Geometry check sheet. Reference: the model listing, model coordinates, mm. Face numbers are marked on the shaded views. A direction names the side the tool comes from. Give positions to 0.01 mm unless a question says otherwise; leave off trailing zeros. Loops run counter-clockwise (first coordinate to the right, second up) from the corner with the lowest first, then second, coordinate; pieces in that order, holes last.
1. Cross-section at C-C, the plane z = 0. Record the cut outline in (x, y).
2. Release check for a two-part mould opening along X. For the marked faces 1, 2 and 3 record: +X half, -X half, draft (parallel to the pull), parting line (faces both ways), or undercut.
3. Cross-section at D-D, the plane y = 52. Record the cut outline in (x, z), plus the area to 3 significant figures.
4. Tool access check on the marked faces 4, 5, 6 and 7. Record the directions out of +Z, -Z, +X, -X, +Y, -Y that give a thin tool (end or side, any length) a straight path to the whole face; none if there is none.
5. Cross-section at A-A, the plane y = 17. Record the cut outline in (x, z).
6. Cross-section at B-B, the plane x = -76.2. Record the cut outline in (y, z), plus the area to 3 significant figures.
7. Go/stop test with flat-tipped pins: pin 1 Ø8 at (y, z) = (21.5, 15.5) entering from +X; pin 2 Ø10 at (y, z) = (45.5, 15) entering from -X; pin 3 Ø1.5 at (x, y) = (57.5, 8) entering from -Z; pin 4 Ø5 at (x, z) = (-60, 14.5) entering from -Y. Record where each tip stops, or that it passes through.
8. Material ranges on L1, parallel to X at y = 28.5, z = 0; L2, parallel to X at y = 37, z = 0; L3, parallel to Z at x = -76, y = 28, recorded low to high.
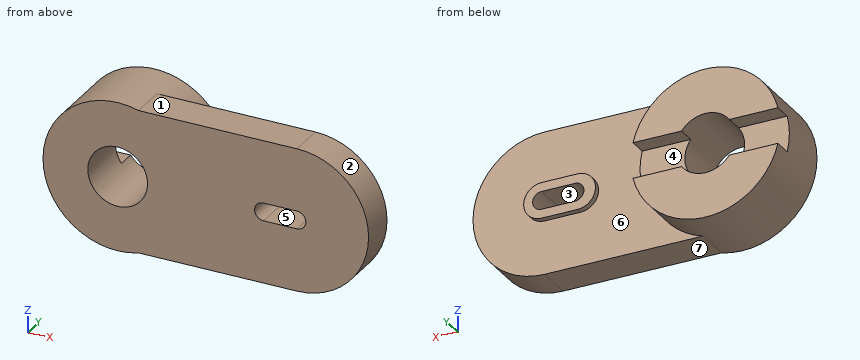
from build123d import *

# Parameters (mm, degrees)
SKETCH2_W           = 152.4
SKETCH2_H           = 121.92
BOSS_EXTRUDE1_DEPTH = 30.48
SKETCH3_R           = 63.5
BOSS_EXTRUDE2_DEPTH = 30.48
SKETCH4_R           = 25.4
CUT_EXTRUDE1_DEPTH  = 60.96
BOSS_EXTRUDE3_DEPTH = 30.48
BOSS_EXTRUDE5_DEPTH = 5.08
CUT_EXTRUDE4_DEPTH  = 35.56
CUT_EXTRUDE5_DEPTH  = 15.24


with BuildPart() as part:
    # Sketch2 → Boss-Extrude1 (new body)
    with BuildSketch(Plane(origin=(0, 0, 0), x_dir=(1, 0, 0), z_dir=(0, 1, 0))):
        Rectangle(SKETCH2_W, SKETCH2_H)
    extrude(amount=BOSS_EXTRUDE1_DEPTH)

    # Sketch3 → Boss-Extrude2 (add, symmetric)
    with BuildSketch(Plane(origin=(0, 30.48, 0), x_dir=(1, 0, 0), z_dir=(0, 1, 0))):
        with Locations(Location((-76.2, 0, 0), (0, 0, 73.739795292))):
            Circle(SKETCH3_R)
    extrude(amount=BOSS_EXTRUDE2_DEPTH, both=True)

    # Sketch4 → Cut-Extrude1 (cut)
    with BuildSketch(Plane(origin=(0, 60.96, 0), x_dir=(1, 0, 0), z_dir=(0, 1, 0))):
        with Locations(Location((-76.2, 0, 0), (0, 0, 270))):
            Circle(SKETCH4_R)
    extrude(amount=-CUT_EXTRUDE1_DEPTH, mode=Mode.SUBTRACT)

    # Sketch5 → Boss-Extrude3 (add)
    with BuildSketch(Plane(origin=(0, 30.48, 0), x_dir=(1, 0, 0), z_dir=(0, 1, 0))):
        with BuildLine():
            Line((76.2, 60.96), (76.2, -60.96))
            ThreePointArc((76.2, -60.96), (137.16, 0), (76.2, 60.96))
        make_face()
    extrude(amount=-BOSS_EXTRUDE3_DEPTH)

    # Sketch6 → Boss-Extrude5 (add)
    with BuildSketch(Plane(origin=(0, 30.48, 0), x_dir=(1, 0, 0), z_dir=(0, 1, 0))):
        with BuildLine():
            Line((76.2, -15.24), (45.597337332, -15.24))
            ThreePointArc((45.597337332, -15.24), (30.357337332, 0), (45.597337332, 15.24))
            Line((45.597337332, 15.24), (76.2, 15.24))
            ThreePointArc((76.2, 15.24), (91.44, 0), (76.2, -15.24))
        make_face()
    extrude(amount=BOSS_EXTRUDE5_DEPTH)

    # Sketch12 → Cut-Extrude4 (cut)
    with BuildSketch(Plane(origin=(0, 35.56, 0), x_dir=(1, 0, 0), z_dir=(0, 1, 0))):
        with BuildLine():
            Line((76.2, -7.62), (47.846010547, -7.62))
            ThreePointArc((47.846010547, -7.62), (40.226010547, 0), (47.846010547, 7.62))
            Line((47.846010547, 7.62), (76.2, 7.62))
            ThreePointArc((76.2, 7.62), (83.82, 0), (76.2, -7.62))
        make_face()
    extrude(amount=-CUT_EXTRUDE4_DEPTH, mode=Mode.SUBTRACT)

    # Sketch14 → Cut-Extrude5 (cut)
    with BuildSketch(Plane(origin=(0, 60.96, 0), x_dir=(1, 0, 0), z_dir=(0, 1, 0))):
        with BuildLine():
            Line((-137.844078386, -15.24), (-14.555921614, -15.24))
            ThreePointArc((-14.555921614, -15.24), (-12.7, 0), (-14.555921614, 15.24))
            Line((-14.555921614, 15.24), (-137.844078386, 15.24))
            ThreePointArc((-137.844078386, 15.24), (-139.7, 0), (-137.844078386, -15.24))
        make_face()
    extrude(amount=-CUT_EXTRUDE5_DEPTH, mode=Mode.SUBTRACT)


solid = part.part
Result:
1. outline: (-139.7, 0) - (-101.6, 0) - (-101.6, 45.72) - (-139.7, 45.72) - close; (-50.8, 0) - (40.23, 0) - (40.23, 35.56) - (30.36, 35.56) - (30.36, 30.48) - (-12.7, 30.48) - (-12.7, 45.72) - (-50.8, 45.72) - close; (83.82, 0) - (137.16, 0) - (137.16, 30.48) - (91.44, 30.48) - (91.44, 35.56) - (83.82, 35.56) - close
2. face 1: draft
2. face 2: +X half
2. face 3: undercut
3. outline: (-137.84, -15.24) arc R63.5 ccw to (-14.56, -15.24) - (-55.88, -15.24) arc R25.4 cw to (-96.52, -15.24) - close; (-137.84, 15.24) - (-96.52, 15.24) arc R25.4 cw to (-55.88, 15.24) - (-14.56, 15.24) arc R63.5 ccw to start
3. area: 8,260 mm2
4. face 4: +X, -X, +Y
4. face 5: +Y, -Y
4. face 6: +Y
4. face 7: -Z, +X, +Y, -Y
5. outline: (-58.42, -60.96) - (76.2, -60.96) arc R60.96 ccw to (76.2, 60.96) - (-58.42, 60.96) arc R63.5 ccw (long way) to start; hole circle Ø50.8 at (-76.2, 0); hole (47.85, -7.62) - (76.2, -7.62) arc R7.62 ccw to (76.2, 7.62) - (47.85, 7.62) arc R7.62 ccw to start
6. outline: (0, -63.5) - (60.96, -63.5) - (60.96, -25.4) - (0, -25.4) - close; (0, 25.4) - (60.96, 25.4) - (60.96, 63.5) - (0, 63.5) - close
6. area: 4,650 mm2
7. pin 1: stops at x = 136.07
7. pin 2: stops at x = -138.91
7. pin 3: stops at z = -60.96
7. pin 4: passes through
8. L1: x = -139.7 to -101.6, -50.8 to 40.23, 83.82 to 137.16
8. L2: x = -139.7 to -101.6, -50.8 to -12.7
8. L3: z = -63.5 to -25.4, 25.4 to 63.5
